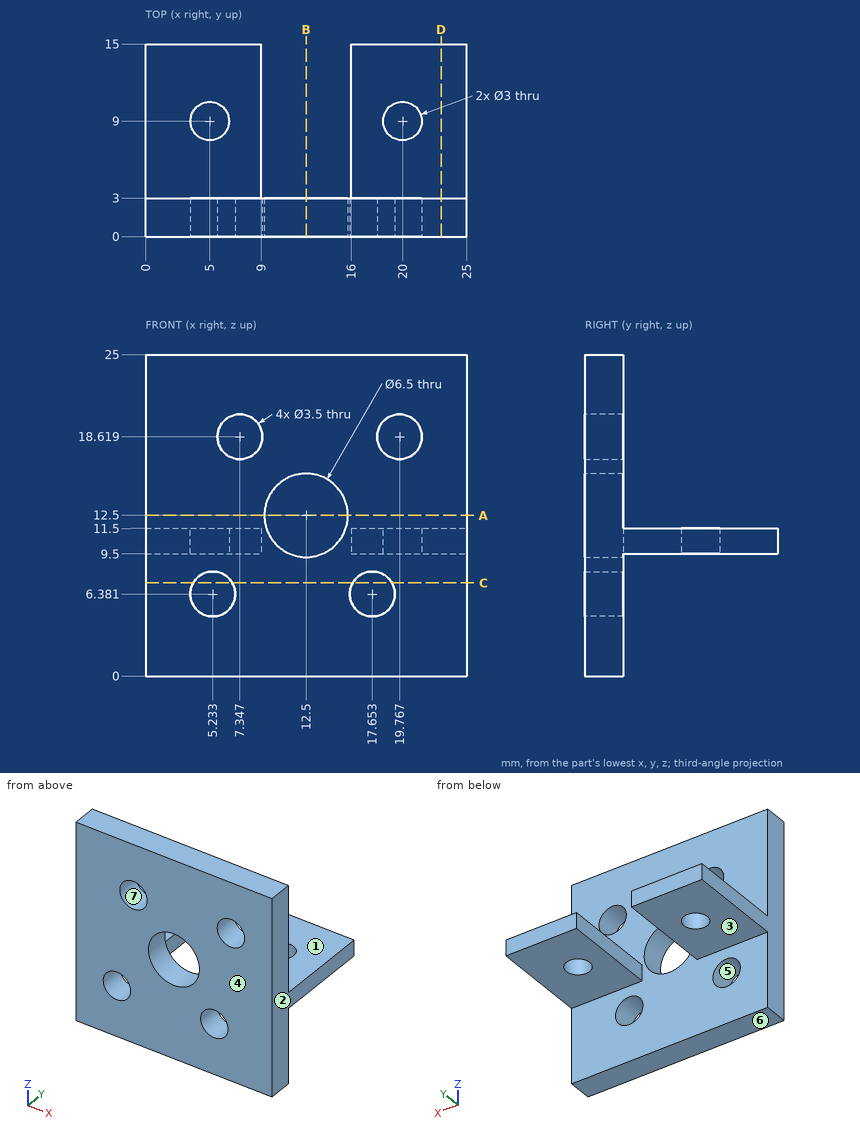
For this review, use the dimensioned drawing (mm, ordinates from the lowest corner) and the shaded views. A direction names the side the tool comes from. Give positions to 0.01 mm unless a question says otherwise; leave off trailing zeros. Order: outer loops, then holes, each group sorted by start corner. A loop starts at its lowest first (then second) coordinate and runs counter-clockwise, first axis right, second up.
1. Mouldability with a two-part tool opening along Z and no side actions: class the marked faces 4, 5, 6 and 7 as +Z half, -Z half, draft (parallel to the pull), parting line (faces both ways), or undercut.
Solution:
face 4: draft
face 5: undercut
face 6: -Z half
face 7: undercut
2. Tool access review of the marked faces 1, 2 and 3: name each direction out of +Z, -Z, +X, -X, +Y, -Y from which nothing blocks a thin tool from reaching the whole face with its end or side.
Solution:
face 1: +Z, +X, -X, +Y
face 2: +Z, -Z, +X, +Y, -Y
face 3: -Z, +X, -X, +Y
3. For pin 1 Ø6 at (x, y) = (10, 10.5) entering from +Z; pin 2 Ø8 at (y, z) = (9.5, 17.5) entering from +X (3 decimals); pin 3 Ø5 at (x, y) = (5, 9) entering from -Z, all flat-tipped, find the tip position at first contact; note any pin that passes through.
Solution:
pin 1: stops at z = 11.5
pin 2: passes through
pin 3: stops at z = 9.5
4. Add section A-A, the plane z = 12.5. State the section outline as (x, y) points.
Solution:
outline: (0, 0) - (9.25, 0) - (9.25, 3) - (0, 3) - close; (15.75, 0) - (25, 0) - (25, 3) - (15.75, 3) - close
5. To check wall thickness, follow L1, parallel to X at y = 0.8, z = 12.5; L2, parallel to Y at x = 5, z = 10.1; L3, parallel to Z at x = 8.5, y = 4.5. State the ranges of each line that lie inside material, in increasing order.
Solution:
L1: x = 0 to 9.25, 15.75 to 25
L2: y = 0 to 7.5, 10.5 to 15
L3: z = 9.5 to 11.5
6. Add section D-D, the plane x = 23. State the section outline as (y, z) points.
Solution:
outline: (0, 0) - (3, 0) - (3, 9.5) - (15, 9.5) - (15, 11.5) - (3, 11.5) - (3, 25) - (0, 25) - close
7. Add section B-B, the plane x = 12.5. State the section outline as (y, z) points.
Solution:
outline: (0, 0) - (3, 0) - (3, 9.25) - (0, 9.25) - close; (0, 15.75) - (3, 15.75) - (3, 25) - (0, 25) - close
8. Add section C-C, the plane z = 7.25. State the section outline as (x, y) points (1 decimal).
Solution:
outline: (0, 0) - (3.7, 0) - (3.7, 3) - (0, 3) - close; (6.8, 0) - (16.1, 0) - (16.1, 3) - (6.8, 3) - close; (19.2, 0) - (25, 0) - (25, 3) - (19.2, 3) - close
